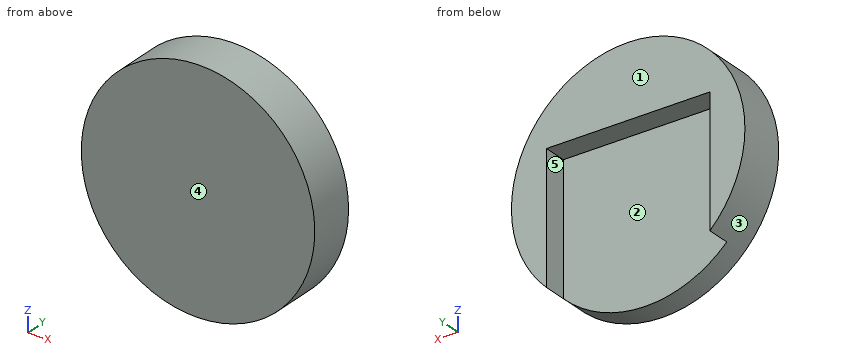
from build123d import *

# Parameters (mm, degrees)
SKETCH1_R           = 50
BOSS_EXTRUDE1_DEPTH = 20
SKETCH2_W           = 70
SKETCH2_H           = 55
CUT_EXTRUDE1_DEPTH  = 10
CUT_EXTRUDE3_START  = -10
CUT_EXTRUDE3_DEPTH  = 10


with BuildPart() as part:
    # Sketch1 → Boss-Extrude1 (new body)
    with BuildSketch(Plane(origin=(0, 0, 0), x_dir=(1, 0, 0), z_dir=(0, 1, 0))):
        with Locations(Location((0, 0, 0), (0, 0, 270))):
            Circle(SKETCH1_R)
    extrude(amount=BOSS_EXTRUDE1_DEPTH)

    # Sketch2 → Cut-Extrude1 (cut)
    with BuildSketch(Plane(origin=(0, 20, 0), x_dir=(1, 0, 0), z_dir=(0, 1, 0))):
        with Locations((-0.015145616, 8.297810168)):
            Rectangle(SKETCH2_W, SKETCH2_H)
    extrude(amount=-CUT_EXTRUDE1_DEPTH, mode=Mode.SUBTRACT)

    # Sketch3 → Cut-Extrude3 (cut)
    with BuildSketch(Plane(origin=(0, 20, 0), x_dir=(1, 0, 0), z_dir=(0, 1, 0)).offset(CUT_EXTRUDE3_START)):
        with BuildLine():
            Line((-35.015145616, 35.692290169), (34.984854384, 35.72198152))
            ThreePointArc((34.984854384, 35.72198152), (-0.021208106, 49.999995502), (-35.015145616, 35.692290169))
        make_face()
    extrude(amount=CUT_EXTRUDE3_DEPTH, mode=Mode.SUBTRACT)


solid = part.part
Source: CAD feature listing. Evaluate the final solid. Frame: model axes, mm. Face numbers are marked on the shaded views. A direction names the side the tool comes from. Give positions to 0.01 mm unless a question says otherwise; leave off trailing zeros. Write each loop counter-clockwise with the first axis right and the second up, starting at its lowest first coordinate (ties: lowest second). Pieces come first, ordered by that corner, then holes. Notation, with made-up numbers: M 84,-6.75 L 106,-6.75 A12 cw 106,12.25 Z; hole C -39.5,45 d3. An arc over 180 degrees is marked long. Return JSON: item names as keys, results as strings. Group by question number.
1) Cut plane D-D, the plane z = -14. Output: boundary loops of the cut face in (x, y).
2) Set-up query: the marked faces 4 and 5. Return all of +Z, -Z, +X, -X, +Y, -Y with unobstructed straight access to the full face (end or side cutting, diameter ignored); none if empty.
3) Cut plane B-B, the plane x = 0. Output: boundary loops of the cut face in (y, z).
4) Cut plane C-C, the plane y = 5. Output: boundary loops of the cut face in (x, z), then the cut area to 3 significant figures.
5) Cut plane A-A, the plane z = 0. Output: boundary loops of the cut face in (x, y).
6) Draft query along X for the marked faces 1, 2 and 3. Return one class per face: released by +X, released by -X, zero draft, split by the parting line, or undercut.
7) First-contact query: pin 1 Ø10 at (y, z) = (16, -35.5) entering from +X; pin 2 Ø2 at (x, y) = (-18, 12) entering from -Z; pin 3 Ø12 at (y, z) = (7, 6.5) entering from +X. Flat tips, straight axial feed; report the tip coordinate or a pass-through.
8) Ray query, L1, parallel to Y at x = 5, z = -30; L2, parallel to X at y = 18, z = -17.5; L3, parallel to X at y = 13, z = -12. Return the intervals inside material, ascending.
Data:
{
 "1": {"outline": "M -48,0 L 48,0 L 48,20 L 34.98,20 L 34.98,10 L -35.02,10 L -35.02,20 L -48,20 Z"},
 "2": {"face 4": "+Z, -Z, +X, -X, -Y", "face 5": "-Z, +Y"},
 "3": {"outline": "M 0,-50 L 10,-50 L 10,19.2 L 20,19.2 L 20,50 L 0,50 Z"},
 "4": {"outline": "C 0,0 d100", "area": "7,850 mm²"},
 "5": {"outline": "M -50,0 L 50,0 L 50,20 L 34.98,20 L 34.98,10 L -35.02,10 L -35.02,20 L -50,20 Z"},
 "6": {"face 1": "zero draft", "face 2": "undercut", "face 3": "split by the parting line"},
 "7": {"pin 1": "stops at x = 39.62", "pin 2": "stops at z = 19.2", "pin 3": "stops at x = 50"},
 "8": {"L1": "y = 0 to 10", "L2": "x = -46.84 to -35.02, 34.98 to 46.84", "L3": "x = -48.54 to -35.02, 34.98 to 48.54"}
}
